from build123d import *

# Parameters (mm, degrees)
SKETCH_1_R               = 60
SKETCH_1_R_2             = 3.95
SKETCH_1_R_3             = 9
SKETCH_1_R_4             = 1.25
EXTRUDE_1_DEPTH          = 3
CUT_EXTRUDE_2_DEPTH      = 85.905830189
PATTERN_CIRCULAR_1_COUNT = 8
CUT_EXTRUDE_3_DEPTH      = 85.905830189
PATTERN_CIRCULAR_2_COUNT = 4
PATTERN_CIRCULAR_2_ANGLE = 135
PATTERN_CIRCULAR_3_COUNT = 4
PATTERN_CIRCULAR_3_ANGLE = 135
CUT_EXTRUDE_6_DEPTH      = 85.905830189


with BuildPart() as part:
    # 草图1 → 凸台-拉伸1 (new body)
    with BuildSketch(Plane.XY):
        Circle(SKETCH_1_R)
        Circle(SKETCH_1_R_2, mode=Mode.SUBTRACT)
        with Locations((23.263813101, 23.263813101)):
            Circle(SKETCH_1_R_3, mode=Mode.SUBTRACT)
        with Locations((0, 55)):
            Circle(SKETCH_1_R_4, mode=Mode.SUBTRACT)
        with Locations(Location((0, -55, 0), (0, 0, 180))):
            Circle(SKETCH_1_R_4, mode=Mode.SUBTRACT)
        with Locations((-55, 0)):
            Circle(SKETCH_1_R_4, mode=Mode.SUBTRACT)
        with Locations(Location((55, 0, 0), (0, 0, 180))):
            Circle(SKETCH_1_R_4, mode=Mode.SUBTRACT)
    extrude(amount=EXTRUDE_1_DEPTH)

    # 草图2 → 切除-拉伸2 (cut, through all)
    with BuildSketch(Plane(origin=(0, 0, 0), x_dir=(-1, 0, 0), z_dir=(0, 0, -1))):
        with BuildLine():
            Line((5.142803301, -9.672206274), (10.317699056, -19.404769676))
            ThreePointArc((10.317699056, -19.404769676), (10.930090319, -19.898002259), (11.709766951, -19.795993482))
            ThreePointArc((11.709766951, -19.795993482), (16.263455967, -16.263455967), (19.795993482, -11.709766951))
            ThreePointArc((19.795993482, -11.709766951), (19.898002259, -10.930090319), (19.404769676, -10.317699056))
            Line((19.404769676, -10.317699056), (9.672206274, -5.142803301))
            ThreePointArc((9.672206274, -5.142803301), (8.954179293, -5.057133217), (8.366122465, -5.477955358))
            ThreePointArc((8.366122465, -5.477955358), (7.071067812, -7.071067812), (5.477955358, -8.366122465))
            ThreePointArc((5.477955358, -8.366122465), (5.057133217, -8.954179293), (5.142803301, -9.672206274))
        make_face()
    cut_extrude_2 = extrude(amount=-CUT_EXTRUDE_2_DEPTH, mode=Mode.SUBTRACT)

    # 阵列(圆周)1: 切除-拉伸2 ×8 about axis
    pattern_circular_1_axis = Axis((0, 0, 0), (0, 0, 1))
    for i in range(1, PATTERN_CIRCULAR_1_COUNT):
        add(cut_extrude_2.rotate(pattern_circular_1_axis, i * 360 / PATTERN_CIRCULAR_1_COUNT), mode=Mode.SUBTRACT)

    # 草图3 → 切除-拉伸3 (cut, through all)
    with BuildSketch(Plane(origin=(0, 0, 0), x_dir=(-1, 0, 0), z_dir=(0, 0, -1))):
        with BuildLine():
            Line((14.546044354, -27.357130582), (22.060168507, -41.489142742))
            ThreePointArc((22.060168507, -41.489142742), (22.660934973, -41.979032326), (23.431267506, -41.89243014))
            ThreePointArc((23.431267506, -41.89243014), (33.941125497, -33.941125497), (41.89243014, -23.431267506))
            ThreePointArc((41.89243014, -23.431267506), (41.979032326, -22.660934973), (41.489142742, -22.060168507))
            Line((41.489142742, -22.060168507), (27.357130582, -14.546044354))
            ThreePointArc((27.357130582, -14.546044354), (26.610751634, -14.468095334), (26.02031518, -14.931282529))
            ThreePointArc((26.02031518, -14.931282529), (21.213203436, -21.213203436), (14.931282529, -26.02031518))
            ThreePointArc((14.931282529, -26.02031518), (14.468095334, -26.610751634), (14.546044354, -27.357130582))
        make_face()
    cut_extrude_3 = extrude(amount=-CUT_EXTRUDE_3_DEPTH, mode=Mode.SUBTRACT)

    # 阵列(圆周)2: 切除-拉伸3 ×4 about axis
    pattern_circular_2_axis = Axis((0, 0, 0), (0, 0, 1))
    for i in range(1, PATTERN_CIRCULAR_2_COUNT):
        add(cut_extrude_3.rotate(pattern_circular_2_axis, i * PATTERN_CIRCULAR_2_ANGLE / (PATTERN_CIRCULAR_2_COUNT - 1)), mode=Mode.SUBTRACT)

    # 阵列(圆周)3: 切除-拉伸3 ×4 about axis
    pattern_circular_3_axis = Axis((0, 0, 0), (0, 0, -1))
    for i in range(1, PATTERN_CIRCULAR_3_COUNT):
        add(cut_extrude_3.rotate(pattern_circular_3_axis, i * PATTERN_CIRCULAR_3_ANGLE / (PATTERN_CIRCULAR_3_COUNT - 1)), mode=Mode.SUBTRACT)

    # 草图4 → 切除-拉伸6 (cut, through all)
    with BuildSketch(Plane(origin=(0, 0, 0), x_dir=(-1, 0, 0), z_dir=(0, 0, -1))):
        with BuildLine():
            Line((-47.86625238, 20.318018681), (-40.502213552, 17.192169654))
            ThreePointArc((-40.502213552, 17.192169654), (-31.112698372, 31.112698372), (-17.192169654, 40.502213552))
            Line((-17.192169654, 40.502213552), (-20.318018681, 47.86625238))
            ThreePointArc((-20.318018681, 47.86625238), (-36.769552622, 36.769552622), (-47.86625238, 20.318018681))
        make_face()
    extrude(amount=-CUT_EXTRUDE_6_DEPTH, mode=Mode.SUBTRACT)


solid = part.part
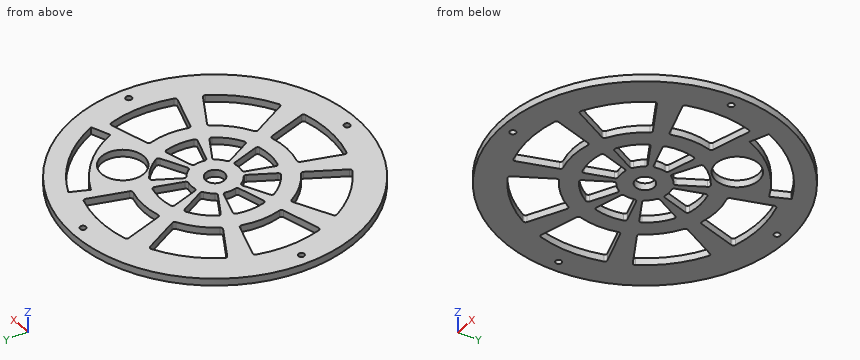
Geometry: final body of the model. Coordinates: model frame, mm. Give positions to 0.01 mm unless a question says otherwise; leave off trailing zeros. Loops run counter-clockwise (first coordinate to the right, second up) from the corner with the lowest first, then second, coordinate; pieces in that order, holes last. Notation, with made-up numbers: (-18.5, 45) - (11.5, 45) arc R16 cw to (11.5, 53) - close; hole circle Ø11 at (70.25, 33.25). An arc over 180 degrees is marked (long way). Answer as CSV lines item,"result". Start each with the question number.
1. Pin query (flat end, axial travel): P1, Ø7, axis at x = 0, y = 0, coming from the +Z side; P2, Ø8, axis at x = -29, y = 11.5, coming from the -Z side; P3, Ø1, axis at y = -8.5, z = 2.5, coming from the +X side. Return the tip coordinate at first contact, or that it passes through.
2. Section B-B, the plane z = 1.55. Give the number of separate pieces and of enclosed holes in the cut face, plus the area to 3 significant figures.
3. Section A-A, the plane x = -18. Return loops of the section in (y, z).
4. Ray query, L1, parallel to Y at x = 21.5, z = 2.8; L2, parallel to Y at x = 22, z = 1.6; L3, parallel to Y at x = -24, z = 1.8. Return the intervals inside material, ascending.
Answers:
1,P1,"passes through"
1,P2,"stops at z = 0"
1,P3,"stops at x = 59.46"
2,separate pieces,"1"
2,enclosed holes,"22"
2,area,"6,770 mm2"
3,outline,"(-57.24, 0) - (-33.85, 0) - (-33.85, 3) - (-57.24, 3) - close; (-24, 0) - (-14.32, 0) - (-14.32, 3) - (-24, 3) - close; (-9.57, 0) - (-5.5, 0) - (-5.5, 3) - (-9.57, 3) - close; (5.5, 0) - (9.57, 0) - (9.57, 3) - (5.5, 3) - close; (14.32, 0) - (24, 0) - (24, 3) - (14.32, 3) - close; (33.85, 0) - (57.24, 0) - (57.24, 3) - (33.85, 3) - close"
4,L1,"y = -56.02 to -40.44, -20.92 to -6.45, 6.45 to 14.44, 32.09 to 38.39, 47.35 to 56.02"
4,L2,"y = -55.82 to -41.38, -20.4 to -6.19, 6.19 to 14.35, 32.17 to 38.11, 47.12 to 55.82"
4,L3,"y = -54.99 to -41.57, -18 to 18, 41.57 to 54.99"
